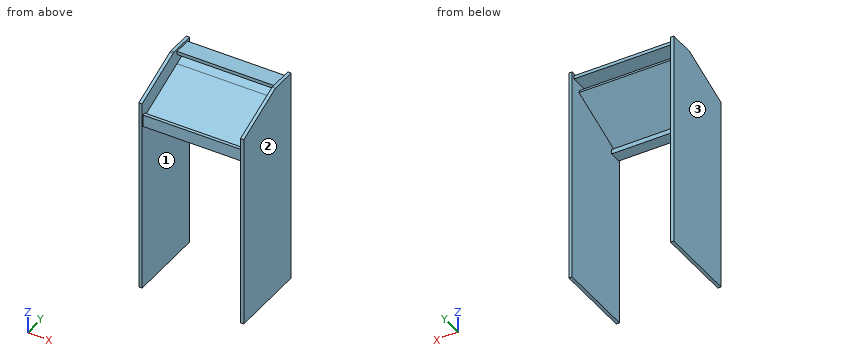
```python
from build123d import *

# Parameters (mm, degrees)
F1_DEPTH  = 19.05
F2_W      = 101.6
F2_H      = 19.05
F3_DEPTH  = 571.5
F5_DEPTH  = 571.5
F6_W      = 571.5
F6_H      = 50.8
F7_DEPTH  = 6.35
F8_DEPTH  = 6.35
F9_W      = 101.6
F9_H      = 19.05
F10_DEPTH = 19.05
F11_DEPTH = 19.05
F12_DEPTH = 50.8


with BuildPart() as f1:
    # F0 (on Right) → F1 (new body)
    with BuildSketch(Plane.YZ):
        with BuildLine():
            Line((228.6, -628.65), (228.6, 628.65))
            Line((228.6, 628.65), (81.28, 628.65))
            ThreePointArc((81.28, 628.65), (76.2986501675, 628.1567491625), (71.5107692308, 626.6961538462))
            Line((71.5107692308, 626.6961538462), (-228.6, 501.65))
            Line((-228.6, 501.65), (-228.6, -628.65))
            Line((-228.6, -628.65), (228.6, -628.65))
        make_face()
    extrude(amount=F1_DEPTH)

    # F2 (on face) → F3 (join)
    with BuildSketch(Plane.YZ.offset(19.05)):
        with Locations((158.75, 606.425)):
            Rectangle(F2_W, F2_H)
    extrude(amount=F3_DEPTH)

    # F4 (on face) → F5 (join)
    with BuildSketch(Plane.YZ.offset(19.05)):
        Polygon((-209.55, 430.2125), (-228.6, 430.2125), (-228.6, 400.05), (-209.55, 407.9875), align=None)
        Polygon((-209.55, 407.9875), (-228.6, 400.05), (-228.6, 379.4125), (-209.55, 387.35), align=None)
        Polygon((-209.55, 387.35), (-228.6, 379.4125), (-209.55, 379.4125), align=None)
        Polygon((107.95, 540.2791666667), (-209.55, 407.9875), (-209.55, 387.35), (162.1692307692, 542.2330128205), (154.8423076923, 559.8176282051), align=None)
    extrude(amount=F5_DEPTH)

    # F6 (on face) → F7 (cut)
    with BuildSketch(Plane.XZ.offset(228.6)):
        with Locations((304.8, 404.8125)):
            Rectangle(F6_W, F6_H)
    extrude(amount=-F7_DEPTH, mode=Mode.SUBTRACT)

    # F8 (add): faces of the model
    f8_faces = [f1.faces().sort_by_distance(p)[0] for p in [
        (304.8, -209.55, 419.1),
        (304.8, -209.55, 383.38125),
    ]]
    extrude(f8_faces, amount=F8_DEPTH)

    # F9 (on face) → F10 (join)
    with BuildSketch(Plane.YZ.offset(590.55)):
        Polygon((228.6, 628.65), (209.55, 628.65), (76.2, 628.65), (-228.6, 501.65), (-228.6, -628.65), (228.6, -628.65), align=None)
        with Locations((158.75, 606.425)):
            Rectangle(F9_W, F9_H, mode=Mode.SUBTRACT)
        with Locations((158.75, 606.425)):
            Rectangle(F9_W, F9_H)
    extrude(amount=F10_DEPTH)

    # F11 (add): a face of the model
    f11_faces = [f1.faces().sort_by_distance(p)[0] for p in [
        (304.8, -212.725, 379.4125),
    ]]
    extrude(f11_faces, amount=F11_DEPTH)

    # F12 (add): a face of the model
    f12_faces = [f1.faces().sort_by_distance(p)[0] for p in [
        (304.8, -203.2, 373.85625),
    ]]
    extrude(f12_faces, amount=F12_DEPTH)


solid = f1.part
```
Source: CAD feature listing. Evaluate the final solid. Frame: model axes, mm. Face numbers are marked on the shaded views. Give positions to 0.01 mm unless a question says otherwise; leave off trailing zeros. Order: outer loops, then holes, each group sorted by start corner. A loop starts at its lowest first (then second) coordinate and runs counter-clockwise, first axis right, second up.
(1) Contact query for flat-ended pins moving along their axis: P1, Ø15, axis at x = 230, y = -213, coming from the +Z side; P2, Ø17, axis at x = 358, y = -168, coming from the +Z side; P3, Ø12, axis at x = 459, y = -143.5, coming from the +Z side. Output: stop coordinate, or through.
(2) Section query D-D (z = 526). Return the cut outline in (x, y), plus the area to 3 significant figures.
(3) Pull-direction query (X, two-part tool) for the marked faces 1, 2 and 3; classes: +X half, -X half, draft (parallel to the pull), parting line (faces both ways), or undercut.
(4) Section query A-A (x = 362). Return the cut outline in (y, z), plus the area to 3 significant figures.
(5) Section query B-B (z = 327). Return the cut outline in (x, y).
(6) Material intervals for line 1 along X through (y, z) = (102.5, 206.5); line 2 along Z through (x, y) = (172, 132); line 3 along Z through (x, y) = (566.5, 194.5), sorted ascending.
(7) Section query C-C (y = 178). Return the cut outline in (x, z).
Outcome:
1. P1: stops at z = 430.21
1. P2: stops at z = 428.84
1. P3: stops at z = 438.01
2. outline: (0, -170.16) - (19.05, -170.16) - (19.05, 73.68) - (590.55, 73.68) - (590.55, -170.16) - (609.6, -170.16) - (609.6, 228.6) - (590.55, 228.6) - (590.55, 123.21) - (19.05, 123.21) - (19.05, 228.6) - (0, 228.6) - close
2. area: 43,500 mm2
3. face 1: undercut
3. face 2: +X half
3. face 3: -X half
4. outline: (-222.25, 360.36) - (-152.4, 360.36) - (-152.4, 387.35) - (-209.55, 387.35) - (162.17, 542.23) - (154.84, 559.82) - (-203.2, 410.63) - (-203.2, 430.21) - (-222.25, 430.21) - close; (107.95, 596.9) - (209.55, 596.9) - (209.55, 615.95) - (107.95, 615.95) - close
4. area: 12,100 mm2
5. outline: (0, -228.6) - (19.05, -228.6) - (19.05, 228.6) - (0, 228.6) - close; (590.55, -228.6) - (609.6, -228.6) - (609.6, 228.6) - (590.55, 228.6) - close
6. line 1: x = 0 to 19.05, 590.55 to 609.6
6. line 2: z = 529.66 to 550.3, 596.9 to 615.95
6. line 3: z = 596.9 to 615.95
7. outline: (0, -628.65) - (19.05, -628.65) - (19.05, 596.9) - (590.55, 596.9) - (590.55, -628.65) - (609.6, -628.65) - (609.6, 628.65) - (590.55, 628.65) - (590.55, 615.95) - (19.05, 615.95) - (19.05, 628.65) - (0, 628.65) - close
